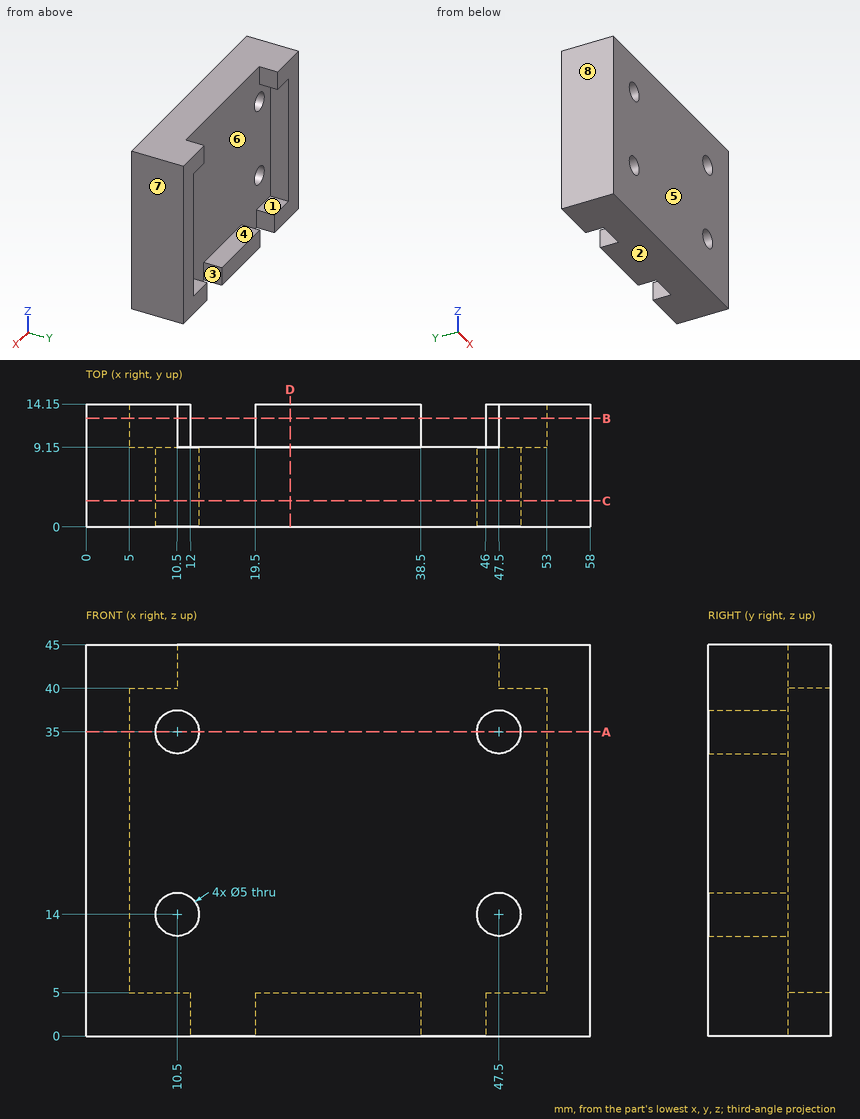
Here's the drawing with two shaded views (mm, measured from the low corner). I have some questions. A direction names the side the tool comes from. Give positions to 0.01 mm unless a question says otherwise; leave off trailing zeros. Loops run counter-clockwise (first coordinate to the right, second up) from the corner with the lowest first, then second, coordinate; pieces in that order, holes last. Notation, with made-up numbers: M -39.5,-38.75 L -25.5,-38.75 A6 ccw -25.5,-33.75 Z; hole C 23.5,-9.5 d4. An arc over 180 degrees is marked long. Answer in a Markdown table with one row per item.
1. If I drill on line 1 along Z through (x, y) = (47.5, 2.5); line 2 along X through (y, z) = (2.5, 35); line 3 along X through (y, z) = (11, 22.5), over which ranges is the centre line in solid material (lowest first)?
Taken from the geometry:
| item | result |
|---|---|
| line 1 | z = 0 to 11.5, 16.5 to 32.5, 37.5 to 45 |
| line 2 | x = 0 to 8, 13 to 45, 50 to 58 |
| line 3 | x = 0 to 5, 53 to 58 |
2. Suppose I cut it at C-C on y = 3. Write out the boundary of the cut face in (x, z).
Taken from the geometry:
| item | result |
|---|---|
| outline | M 0,0 L 58,0 L 58,45 L 0,45 Z; hole C 10.5,14 d5; hole C 10.5,35 d5; hole C 47.5,14 d5; hole C 47.5,35 d5 |
3. Thinking about a two-plate mould opening in X: for the marked faces 5, 6, 7 and 8, which applies, released by +X, released by -X, zero draft, split by the parting line, or undercut?
Taken from the geometry:
| item | result |
|---|---|
| face 5 | zero draft |
| face 6 | undercut |
| face 7 | released by +X |
| face 8 | released by -X |
4. For pin 1 Ø6 at (x, z) = (10.5, 35) entering from +Y; pin 2 Ø6 at (x, z) = (21, 11.5) entering from +Y; pin 3 Ø1 at (y, z) = (1.5, 32) entering from -X; pin 4 Ø1.5 at (x, y) = (29.5, 12) entering from +Z, each with a flat end and sliding along its axis, tell me the tip position at first contact or that it passes through.
Taken from the geometry:
| item | result |
|---|---|
| pin 1 | stops at y = 9.15 |
| pin 2 | stops at y = 9.15 |
| pin 3 | stops at x = 0 |
| pin 4 | stops at z = 5 |
5. Suppose I cut it at B-B on y = 12.5. Write out the boundary of the cut face in (x, z).
Taken from the geometry:
| item | result |
|---|---|
| outline | M 0,0 L 12,0 L 12,5 L 5,5 L 5,40 L 10.5,40 L 10.5,45 L 0,45 Z; M 19.5,0 L 38.5,0 L 38.5,5 L 19.5,5 Z; M 46,0 L 58,0 L 58,45 L 47.5,45 L 47.5,40 L 53,40 L 53,5 L 46,5 Z |
6. Suppose I cut it at D-D on x = 23.5. Write out the boundary of the cut face in (y, z), plus the area to 3 significant figures.
Taken from the geometry:
| item | result |
|---|---|
| outline | M 0,0 L 14.15,0 L 14.15,5 L 9.15,5 L 9.15,45 L 0,45 Z |
| area | 437 mm² |
7. Suppose I cut it at A-A on z = 35. Write out the boundary of the cut face in (x, y), plus the area to 3 significant figures.
Taken from the geometry:
| item | result |
|---|---|
| outline | M 0,0 L 8,0 L 8,9.15 L 5,9.15 L 5,14.15 L 0,14.15 Z; M 13,0 L 45,0 L 45,9.15 L 13,9.15 Z; M 50,0 L 58,0 L 58,14.15 L 53,14.15 L 53,9.15 L 50,9.15 Z |
| area | 489 mm² |
8. Which directions (+Z, -Z, +X, -X, +Y, -Y) give clear straight access to the entire face, cutting with the end or side of a thin tool? Please do the marked faces 1, 2, 3 and 4.
Taken from the geometry:
| item | result |
|---|---|
| face 1 | +Y |
| face 2 | -Z, +X, -X, +Y, -Y |
| face 3 | +Z, -Z, +Y |
| face 4 | +Z, +Y |
